The listing builds one solid part. Answer for the finished solid, in the listing's coordinates (mm). A direction names the side the tool comes from. Round coordinates to 2 decimals unless told otherwise and drop trailing zeros. Write each loop counter-clockwise with the first axis right and the second up, starting at its lowest first coordinate (ties: lowest second). Pieces come first, ordered by that corner, then holes.
(1) Each of these flat-tipped pins is pushed along its axis until it touches: pin 1 Ø6 at (x, z) = (73, 8) entering from -Y; pin 2 Ø1.2 at (y, z) = (-2, 3.5) entering from +X. Where does it stop, or does it pass through?
(2) A cutting plane is placed at A-A, the plane x = 80. Give the vertices of the cut face in (y, z).
(3) The mould has two halves that part along X. Classify faces 1 (the face through (90, 5, 6)), 2 (the face through (64, 2.4, 6)), 3 (the face through (44, 10, 6)): +X half, -X half, draft (parallel to the pull), parting line (faces both ways), or undercut.
(4) For faces 4 (the face through (0, 4, 6)), 5 (the face through (2.5, -2, 6)), 6 (the face through (65, 7.6, 6)), determine the directions among +Z, -Z, +X, -X, +Y, -Y from which every point of the face is accessible in a straight line to the end or side of a thin tool.
(5) A cutting plane is placed at C-C, the plane z = 6.5. Give the vertices of the cut face in (x, y).
(6) A cutting plane is placed at B-B, the plane y = 5. Give the vertices of the cut face in (x, z).
(7) Find the intervals of material crossed by probe 1 along Y at (x, z) = (70.5, 5.25); probe 2 along X at (y, z) = (-2, 6.25); probe 3 along Y at (x, z) = (22, 5), in increasing order.
(8) A cutting plane is placed at D-D, the plane x = 7.5. Give the vertices of the cut face in (y, z).
from build123d import *

# Parameters (mm, degrees)
SKETCH_1_W          = 90
SKETCH_1_H          = 10
EXTRUDE_1_DEPTH     = 12
SKETCH_2_W          = 2.5
SKETCH_2_H          = 12
EXTRUDE_2_DEPTH     = 3
CUT_EXTRUDE_1_DEPTH = 92.345497973
FILLET_1_R          = 0.5


with BuildPart() as part:
    # 草图1 → 凸台-拉伸1 (new body)
    with BuildSketch(Plane.XY):
        with Locations((45, 5)):
            Rectangle(SKETCH_1_W, SKETCH_1_H)
    extrude(amount=EXTRUDE_1_DEPTH)

    # 草图2 → 凸台-拉伸2 (add)
    with BuildSketch(Plane.XZ):
        with Locations((1.25, 6)):
            Rectangle(SKETCH_2_W, SKETCH_2_H)
    extrude(amount=EXTRUDE_2_DEPTH)

    # 草图3 → 切除-拉伸1 (cut, through all)
    with BuildSketch(Plane(origin=(0, 0, 0), x_dir=(-1, 0, 0), z_dir=(0, 0, -1))):
        with BuildLine():
            Line((-82, 7.6), (-47, 7.6))
            ThreePointArc((-47, 7.6), (-44.4, 5), (-47, 2.4))
            Line((-47, 2.4), (-82, 2.4))
            ThreePointArc((-82, 2.4), (-84.6, 5), (-82, 7.6))
        make_face()
    extrude(amount=-CUT_EXTRUDE_1_DEPTH, mode=Mode.SUBTRACT)

    # 圆角1
    fillet_1_edges = [part.edges().sort_by_distance(p)[0] for p in [
        (2.5, 0, 6),
    ]]
    fillet(fillet_1_edges, radius=FILLET_1_R)


solid = part.part
Solutions:
1. pin 1: stops at y = 0
1. pin 2: stops at x = 2.5
2. outline: (0, 0) - (2.4, 0) - (2.4, 12) - (0, 12) - close; (7.6, 0) - (10, 0) - (10, 12) - (7.6, 12) - close
3. face 1: +X half
3. face 2: undercut
3. face 3: draft
4. face 4: +Z, -Z, -X, +Y, -Y
4. face 5: +Z, -Z, +X, -Y
4. face 6: +Z, -Z
5. outline: (0, -3) - (2.5, -3) - (2.5, -0.5) arc R0.5 cw to (3, 0) - (90, 0) - (90, 10) - (0, 10) - close; hole (47, 2.4) - (82, 2.4) arc R2.6 ccw to (82, 7.6) - (47, 7.6) arc R2.6 ccw to start
6. outline: (0, 0) - (44.4, 0) - (44.4, 12) - (0, 12) - close; (84.6, 0) - (90, 0) - (90, 12) - (84.6, 12) - close
7. probe 1: y = 0 to 2.4, 7.6 to 10
7. probe 2: x = 0 to 2.5
7. probe 3: y = 0 to 10
8. outline: (0, 0) - (10, 0) - (10, 12) - (0, 12) - close
